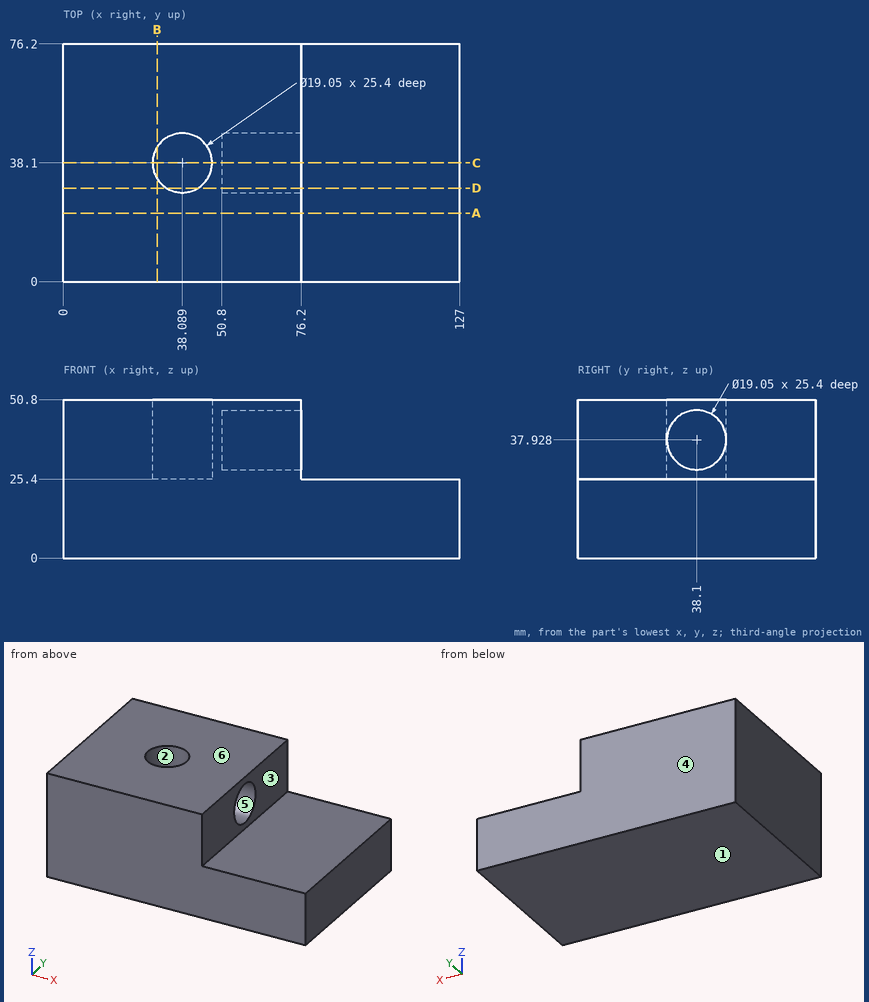
Study the drawing (mm; zero at the part's minimum x, y, z) and answer. A direction names the side the tool comes from. Give positions to 0.01 mm unless a question says otherwise; leave off trailing zeros. Write each loop counter-clockwise with the first axis right and the second up, starting at its lowest first coordinate (ties: lowest second). Pieces come first, ordered by that corner, then holes.
(1) Flat-ended cylindrical pins translate along their axes: pin 1 Ø12 at (y, z) = (9.5, 45) entering from +X; pin 2 Ø9.5 at (y, z) = (36.5, 39) entering from +X; pin 3 Ø8 at (x, y) = (97.5, 42) entering from +Z. Find the tip coordinate at first contact, or state that the pin passes through.
Final values:
pin 1: stops at x = 76.2
pin 2: stops at x = 50.8
pin 3: stops at z = 25.4
(2) Which of the six approach directions +Z, -Z, +X, -X, +Y, -Y give full straight-line access (tool end or side, diameter ignored) to the marked faces 1, 2 and 3?
Final values:
face 1: -Z, +X, -X, +Y, -Y
face 2: +Z
face 3: +Z, +X, +Y, -Y
(3) The part is cut by section D-D on y = 30. Write down the section's boundary in (x, z).
Final values:
outline: (0, 0) - (127, 0) - (127, 25.4) - (76.2, 25.4) - (76.2, 32.92) - (50.8, 32.92) - (50.8, 42.94) - (76.2, 42.94) - (76.2, 50.8) - (43.1, 50.8) - (43.1, 25.4) - (33.08, 25.4) - (33.08, 50.8) - (0, 50.8) - close
(4) The part is cut by section A-A on y = 22. Write down the section's boundary in (x, z).
Final values:
outline: (0, 0) - (127, 0) - (127, 25.4) - (76.2, 25.4) - (76.2, 50.8) - (0, 50.8) - close
(5) The part is cut by section C-C on y = 38.1. Write down the section's boundary in (x, z), plus the area to 3 significant figures.
Final values:
outline: (0, 0) - (127, 0) - (127, 25.4) - (76.2, 25.4) - (76.2, 28.4) - (50.8, 28.4) - (50.8, 47.45) - (76.2, 47.45) - (76.2, 50.8) - (47.61, 50.8) - (47.61, 25.4) - (28.56, 25.4) - (28.56, 50.8) - (0, 50.8) - close
area: 4,190 mm2
(6) The mould has two halves that part along Y. Classify the marked faces 4, 5 and 6: pulls with the +Y half, pulls with the -Y half, needs draft (parallel to the pull), parting line crosses it, or undercut.
Final values:
face 4: pulls with the +Y half
face 5: undercut
face 6: needs draft
(7) The part is cut by section B-B on x = 30. Write down the section's boundary in (y, z), plus the area to 3 significant figures.
Final values:
outline: (0, 0) - (76.2, 0) - (76.2, 50.8) - (43.13, 50.8) - (43.13, 25.4) - (33.07, 25.4) - (33.07, 50.8) - (0, 50.8) - close
area: 3,620 mm2
(8) Straight lines are drawn through the part: line 1 (Z direction, x = 58.25, y = 38.1); line 2 (Z direction, x = 116.5, y = 10); line 3 (X direction, y = 5, z = 27). For each, find the intervals that lie inside material, in ascending order.
Final values:
line 1: z = 0 to 28.4, 47.45 to 50.8
line 2: z = 0 to 25.4
line 3: x = 0 to 76.2
